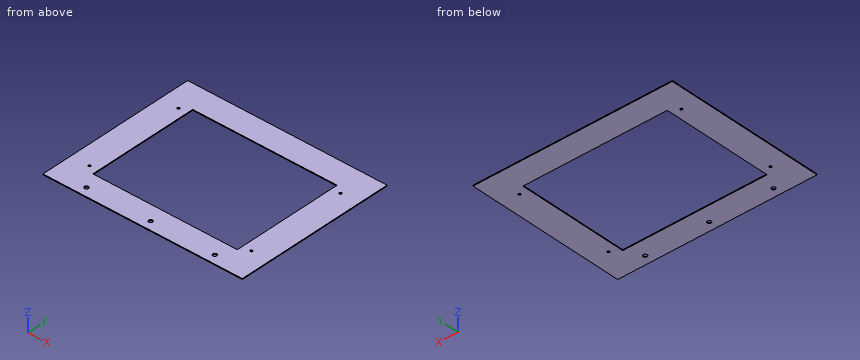
```python
from build123d import *

# Parameters (mm, degrees)
SKETCH_1_W      = 248.5
SKETCH_1_H      = 200
SKETCH_1_R      = 2.5
SKETCH_1_R_2    = 1.5
SKETCH_1_W_2    = 180
SKETCH_1_H_2    = 138
EXTRUDE_1_DEPTH = 0.5


with BuildPart() as part:
    # 스케치1 → 보스-돌출1 (new, symmetric)
    with BuildSketch(Plane.XY):
        with Locations((124.25, 100)):
            Rectangle(SKETCH_1_W, SKETCH_1_H)
        with Locations((124.25, 11)):
            Circle(SKETCH_1_R, mode=Mode.SUBTRACT)
        with Locations((204.25, 11)):
            Circle(SKETCH_1_R, mode=Mode.SUBTRACT)
        with Locations((44.25, 11)):
            Circle(SKETCH_1_R, mode=Mode.SUBTRACT)
        with Locations((225.215, 161.595)):
            Circle(SKETCH_1_R_2, mode=Mode.SUBTRACT)
        with Locations((225.215, 38.405)):
            Circle(SKETCH_1_R_2, mode=Mode.SUBTRACT)
        with Locations(Location((23.285, 38.405, 0), (0, 0, 180))):
            Circle(SKETCH_1_R_2, mode=Mode.SUBTRACT)
        with Locations(Location((23.285, 161.595, 0), (0, 0, 180))):
            Circle(SKETCH_1_R_2, mode=Mode.SUBTRACT)
        with Locations((124.25, 100)):
            Rectangle(SKETCH_1_W_2, SKETCH_1_H_2, mode=Mode.SUBTRACT)
    extrude(amount=EXTRUDE_1_DEPTH, both=True)


solid = part.part
```
Source: CAD feature listing. Evaluate the final solid. Frame: model axes, mm. Round coordinates to 2 decimals unless told otherwise and drop trailing zeros. Loops run counter-clockwise (first coordinate to the right, second up) from the corner with the lowest first, then second, coordinate; pieces in that order, holes last. Notation, with made-up numbers: M 47.25,66 L 79.25,66 A23 ccw 79.25,102 Z; hole C 74.25,64 d7. An arc over 180 degrees is marked long. Use a Markdown table: item, result. Add a question column.
1. Ray query, line 1 along Y through (x, z) = (204.25, 0.05); line 2 along Y through (x, z) = (140, 0.05); line 3 along X through (y, z) = (164.5, 0.25). Return the intervals inside material, ascending. Write a range as [from, to].
2. Cut plane A-A, the plane y = 116. Output: boundary loops of the cut face in (x, z).
3. Cut plane B-B, the plane x = 157. Output: boundary loops of the cut face in (y, z), and give its area (3 significant figures).
4. Cut plane C-C, the plane z = 0.35. State how many separate pieces and enclosed holes the cut face has, and give its area (3 significant figures).
5. Contact query for a flat-ended pin moving along its axis: pin 1 (5 mm diameter, centred on x = 225.215, y = 38.405, fed in from +Z). Output: stop coordinate, or through.
Solution:
| question | item | result |
|---|---|---|
| 1 | line 1 | y = [0, 8.5], [13.5, 31], [169, 200] |
| 1 | line 2 | y = [0, 31], [169, 200] |
| 1 | line 3 | x = [0, 34.25], [214.25, 248.5] |
| 2 | outline | M 0,-0.5 L 34.25,-0.5 L 34.25,0.5 L 0,0.5 Z; M 214.25,-0.5 L 248.5,-0.5 L 248.5,0.5 L 214.25,0.5 Z |
| 3 | outline | M 0,-0.5 L 31,-0.5 L 31,0.5 L 0,0.5 Z; M 169,-0.5 L 200,-0.5 L 200,0.5 L 169,0.5 Z |
| 3 | area | 62.0 mm2 |
| 4 | separate pieces | 1 |
| 4 | enclosed holes | 8 |
| 4 | area | 24,800 mm2 |
| 5 | pin 1 | stops at z = 0.5 |
